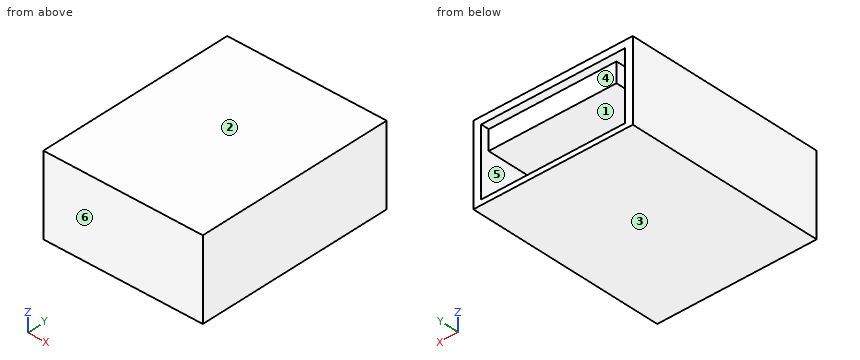
```python
from build123d import *

# Parameters (mm, degrees)
F0_W     = 12
F0_H     = 15
F1_DEPTH = 6
F2_W     = 10.816304
F2_H     = 5.077495
F3_DEPTH = 14
F4_W     = 9.618904
F4_H     = 1.474254
F5_DEPTH = 14


with BuildPart() as f1:
    # F0 (on Top) → F1 (new body)
    with BuildSketch(Plane.XY):
        Rectangle(F0_W, F0_H)
    extrude(amount=F1_DEPTH)

    # F2 (on face) → F3 (cut)
    with BuildSketch(Plane(origin=(0, 7.5, 0), x_dir=(-1, 0, 0), z_dir=(0, 1, 0))):
        with Locations((0, 2.921203)):
            Rectangle(F2_W, F2_H)
    extrude(amount=-F3_DEPTH, mode=Mode.SUBTRACT)

    # F4 (on face) → F5 (join)
    with BuildSketch(Plane(origin=(0, -6.5, 0), x_dir=(-1, 0, 0), z_dir=(0, 1, 0))):
        with Locations((-0.038077, 4.130425)):
            Rectangle(F4_W, F4_H)
    extrude(amount=F5_DEPTH)


solid = f1.part
```
Can you work these out from the model? Positions are in its coordinate system, mm. Face numbers are marked on the shaded views. A direction names the side the tool comes from. Round coordinates to 2 decimals unless told otherwise and drop trailing zeros. Loops run counter-clockwise (first coordinate to the right, second up) from the corner with the lowest first, then second, coordinate; pieces in that order, holes last. Notation, with made-up numbers: M 15,37 L 74,37 A26 ccw 74,53 Z; hole C 85,-15.5 d10. An arc over 180 degrees is marked long. Write item = value, one per line. Start each with the question number.
(1) Suppose I cut it at A-A on y = 0. Write out the boundary of the cut face in (x, z).
(2) Suppose I cut it at B-B on z = 1.1. Write out the boundary of the cut face in (x, y).
(3) Suppose I cut it at D-D on z = 4.6. Write out the boundary of the cut face in (x, y).
(4) If we mould it in two halves opening along Z, with no side actions, what happens to the marked faces 1, 2, 3 and 4? For each: released by +Z, released by -Z, zero draft, split by the parting line, or undercut.
(5) Suppose I cut it at C-C on x = -0.75. Write out the boundary of the cut face in (y, z), plus the area to 3 significant figures.
(6) I need wall thicknesses on line 1 along Z through (x, y) = (4.25, 0.5); line 2 along X through (y, z) = (3, 4.4); line 3 along Z through (x, y) = (5, 6.5). Which ranges of each line are inside material? Lowest first, please.
(7) Which directions (+Z, -Z, +X, -X, +Y, -Y) give clear straight access to the entire face, cutting with the end or side of a thin tool? Please do the marked faces 5 and 6.
Answer block:
q1.outline = M -6,0 L 6,0 L 6,6 L -6,6 Z; M -4.77,3.39 L 4.85,3.39 L 4.85,4.87 L -4.77,4.87 Z; hole M -5.41,0.38 L 5.41,0.38 L 5.41,5.46 L -5.41,5.46 Z
q2.outline = M -6,-7.5 L 6,-7.5 L 6,7.5 L 5.41,7.5 L 5.41,-6.5 L -5.41,-6.5 L -5.41,7.5 L -6,7.5 Z
q3.outline = M -6,-7.5 L 6,-7.5 L 6,7.5 L 5.41,7.5 L 5.41,-6.5 L 4.85,-6.5 L 4.85,7.5 L -4.77,7.5 L -4.77,-6.5 L -5.41,-6.5 L -5.41,7.5 L -6,7.5 Z
q4.face_1 = undercut
q4.face_2 = released by +Z
q4.face_3 = released by -Z
q4.face_4 = zero draft
q5.outline = M -7.5,0 L 7.5,0 L 7.5,0.38 L -6.5,0.38 L -6.5,3.39 L 7.5,3.39 L 7.5,4.87 L -6.5,4.87 L -6.5,5.46 L 7.5,5.46 L 7.5,6 L -7.5,6 Z
q5.area = 39.6 mm²
q6.line_1 = 0 to 0.38, 3.39 to 4.87, 5.46 to 6
q6.line_2 = -6 to -5.41, -4.77 to 4.85, 5.41 to 6
q6.line_3 = 0 to 0.38, 5.46 to 6
q7.face_5 = +Y
q7.face_6 = +Z, -Z, +X, -X, -Y
